Input: part model. Units: mm. Frame: model coordinates. A direction names the side the tool comes from. Coordinates: 2 decimals unless noted, no trailing zeros. Write each loop counter-clockwise with the first axis right and the second up, starting at its lowest first coordinate (ties: lowest second). Pieces come first, ordered by that corner, then holes.
1) Section query B-B (x = -119). Output: boundary loops of the cut face in (y, z).
2) Set-up query: faces 1 (the flat face through (-35, 19, -50)), 2 (the flat face through (-83, 7, 23)), 3 (the flat face through (-240, 19, -25.991)), 4 (the flat face through (-240, 19, 124.009)). Return all of +Z, -Z, +X, -X, +Y, -Y with unobstructed straight access to the full face (end or side cutting, diameter ignored); none if empty.
3) Pin query (flat end, axial travel): pin 1 Ø1.5 at (x, y) = (-18, 20) entering from +Z; pin 2 Ø1.6 at (y, z) = (6.5, -4) entering from +X; pin 3 Ø7.5 at (y, z) = (25.5, -47) entering from -X. Return the tip coordinate at first contact, or that it passes through.
4) Draft query along Y for faces 5 (the flat face through (-240, 32, 99)), 6 (the flat face through (-243, 7, 73)), 7 (the flat face through (-80, 19, 75.261)). Return one class per face: pulls with the +Y half, pulls with the -Y half, needs draft (parallel to the pull), parting line crosses it, or undercut.
5) Section query A-A (y = 16.5). State how many separate pieces and enclosed holes the cut face has, then the cut area to 3 significant figures.
6) Line query: L1, parallel to X at y = 27.5, z = 55; L2, parallel to Z at x = 5.5, y = 20.5. Output: solid intervals per line, ascending.
from build123d import *

# Parameters (mm, degrees)
SKETCH1_W                  = 80
SKETCH1_H                  = 270
BOSS_EXTRUDE1_DEPTH        = 5
SKETCH2_W                  = 65
SKETCH2_H                  = 45
BOSS_EXTRUDE3_DEPTH        = 2
LPATTERN1_COUNT            = 5
LPATTERN1_PITCH            = 50
SKETCH3_W                  = 70
SKETCH3_H                  = 48.748964222
BOSS_EXTRUDE8_DEPTH        = 25
LPATTERN5_COUNT            = 5
LPATTERN5_PITCH            = 50
LPATTERN6_COUNT            = 4
LPATTERN6_PITCH            = 80
LPATTERN6_COPY_1_SKETCH_W  = 65
LPATTERN6_COPY_1_SKETCH_H  = 45
LPATTERN6_COPY_1_DEPTH     = 2
LPATTERN6_COPY_2_SKETCH_W  = 65
LPATTERN6_COPY_2_SKETCH_H  = 45
LPATTERN6_COPY_2_DEPTH     = 2
LPATTERN6_COPY_3_SKETCH_W  = 65
LPATTERN6_COPY_3_SKETCH_H  = 45
LPATTERN6_COPY_3_DEPTH     = 2
LPATTERN6_COPY_4_SKETCH_W  = 65
LPATTERN6_COPY_4_SKETCH_H  = 45
LPATTERN6_COPY_4_DEPTH     = 2
LPATTERN6_COPY_5_SKETCH_W  = 65
LPATTERN6_COPY_5_SKETCH_H  = 45
LPATTERN6_COPY_5_DEPTH     = 2
LPATTERN6_COPY_6_SKETCH_W  = 65
LPATTERN6_COPY_6_SKETCH_H  = 45
LPATTERN6_COPY_6_DEPTH     = 2
LPATTERN6_COPY_7_SKETCH_W  = 65
LPATTERN6_COPY_7_SKETCH_H  = 45
LPATTERN6_COPY_7_DEPTH     = 2
LPATTERN6_COPY_8_SKETCH_W  = 65
LPATTERN6_COPY_8_SKETCH_H  = 45
LPATTERN6_COPY_8_DEPTH     = 2
LPATTERN6_COPY_9_SKETCH_W  = 65
LPATTERN6_COPY_9_SKETCH_H  = 45
LPATTERN6_COPY_9_DEPTH     = 2
LPATTERN6_COPY_10_SKETCH_W = 65
LPATTERN6_COPY_10_SKETCH_H = 45
LPATTERN6_COPY_10_DEPTH    = 2
LPATTERN6_COPY_11_SKETCH_W = 65
LPATTERN6_COPY_11_SKETCH_H = 45
LPATTERN6_COPY_11_DEPTH    = 2
LPATTERN6_COPY_12_SKETCH_W = 65
LPATTERN6_COPY_12_SKETCH_H = 45
LPATTERN6_COPY_12_DEPTH    = 2
LPATTERN6_COPY_13_SKETCH_W = 70
LPATTERN6_COPY_13_SKETCH_H = 48.748964222
LPATTERN6_COPY_13_DEPTH    = 25
LPATTERN6_COPY_14_SKETCH_W = 70
LPATTERN6_COPY_14_SKETCH_H = 48.748964222
LPATTERN6_COPY_14_DEPTH    = 25
LPATTERN6_COPY_15_SKETCH_W = 70
LPATTERN6_COPY_15_SKETCH_H = 48.748964222
LPATTERN6_COPY_15_DEPTH    = 25
LPATTERN6_COPY_16_SKETCH_W = 70
LPATTERN6_COPY_16_SKETCH_H = 48.748964222
LPATTERN6_COPY_16_DEPTH    = 25
LPATTERN6_COPY_17_SKETCH_W = 70
LPATTERN6_COPY_17_SKETCH_H = 48.748964222
LPATTERN6_COPY_17_DEPTH    = 25
LPATTERN6_COPY_18_SKETCH_W = 70
LPATTERN6_COPY_18_SKETCH_H = 48.748964222
LPATTERN6_COPY_18_DEPTH    = 25
LPATTERN6_COPY_19_SKETCH_W = 70
LPATTERN6_COPY_19_SKETCH_H = 48.748964222
LPATTERN6_COPY_19_DEPTH    = 25
LPATTERN6_COPY_20_SKETCH_W = 70
LPATTERN6_COPY_20_SKETCH_H = 48.748964222
LPATTERN6_COPY_20_DEPTH    = 25
LPATTERN6_COPY_21_SKETCH_W = 70
LPATTERN6_COPY_21_SKETCH_H = 48.748964222
LPATTERN6_COPY_21_DEPTH    = 25
LPATTERN6_COPY_22_SKETCH_W = 70
LPATTERN6_COPY_22_SKETCH_H = 48.748964222
LPATTERN6_COPY_22_DEPTH    = 25
LPATTERN6_COPY_23_SKETCH_W = 70
LPATTERN6_COPY_23_SKETCH_H = 48.748964222
LPATTERN6_COPY_23_DEPTH    = 25
LPATTERN6_COPY_24_SKETCH_W = 70
LPATTERN6_COPY_24_SKETCH_H = 48.748964222
LPATTERN6_COPY_24_DEPTH    = 25


with BuildPart() as part:
    # Sketch1 → Boss-Extrude1 (new body)
    with BuildSketch(Plane(origin=(0, 0, 0), x_dir=(1, 0, 0), z_dir=(0, 1, 0))):
        Rectangle(SKETCH1_W, SKETCH1_H)
    boss_extrude1 = extrude(amount=BOSS_EXTRUDE1_DEPTH)

    # Sketch2 → Boss-Extrude3 (add)
    with BuildSketch(Plane(origin=(0, 5, 0), x_dir=(1, 0, 0), z_dir=(0, 1, 0))):
        with Locations((0, -100)):
            Rectangle(SKETCH2_W, SKETCH2_H)
    boss_extrude3 = extrude(amount=BOSS_EXTRUDE3_DEPTH)

    # LPattern1: Boss-Extrude3 ×5
    with Locations(*[(0, 0, -i * LPATTERN1_PITCH) for i in range(1, LPATTERN1_COUNT)]):
        add(boss_extrude3)

    # Sketch3 → Boss-Extrude8 (add)
    with BuildSketch(Plane(origin=(0, 7, 0), x_dir=(1, 0, 0), z_dir=(0, 1, 0))):
        with Locations((0, -99.635002086)):
            Rectangle(SKETCH3_W, SKETCH3_H)
    boss_extrude8 = extrude(amount=BOSS_EXTRUDE8_DEPTH)

    # LPattern5: Boss-Extrude8 ×5
    with Locations(*[(0, 0, -i * LPATTERN5_PITCH) for i in range(1, LPATTERN5_COUNT)]):
        add(boss_extrude8)

    # LPattern6: Boss-Extrude1, Boss-Extrude3, Boss-Extrude8 ×4
    with Locations(*[(-i * LPATTERN6_PITCH, 0, 0) for i in range(1, LPATTERN6_COUNT)]):
        add(boss_extrude1)
        add(boss_extrude3)
        add(boss_extrude8)

    # LPattern6 copy 1 sketch → LPattern6 copy 1 (add)
    with BuildSketch(Plane(origin=(-80, 5, -50), x_dir=(1, 0, 0), z_dir=(0, 1, 0))):
        with Locations((0, -100)):
            Rectangle(LPATTERN6_COPY_1_SKETCH_W, LPATTERN6_COPY_1_SKETCH_H)
    extrude(amount=LPATTERN6_COPY_1_DEPTH)

    # LPattern6 copy 2 sketch → LPattern6 copy 2 (add)
    with BuildSketch(Plane(origin=(-160, 5, -50), x_dir=(1, 0, 0), z_dir=(0, 1, 0))):
        with Locations((0, -100)):
            Rectangle(LPATTERN6_COPY_2_SKETCH_W, LPATTERN6_COPY_2_SKETCH_H)
    extrude(amount=LPATTERN6_COPY_2_DEPTH)

    # LPattern6 copy 3 sketch → LPattern6 copy 3 (add)
    with BuildSketch(Plane(origin=(-240, 5, -50), x_dir=(1, 0, 0), z_dir=(0, 1, 0))):
        with Locations((0, -100)):
            Rectangle(LPATTERN6_COPY_3_SKETCH_W, LPATTERN6_COPY_3_SKETCH_H)
    extrude(amount=LPATTERN6_COPY_3_DEPTH)

    # LPattern6 copy 4 sketch → LPattern6 copy 4 (add)
    with BuildSketch(Plane(origin=(-80, 5, -100), x_dir=(1, 0, 0), z_dir=(0, 1, 0))):
        with Locations((0, -100)):
            Rectangle(LPATTERN6_COPY_4_SKETCH_W, LPATTERN6_COPY_4_SKETCH_H)
    extrude(amount=LPATTERN6_COPY_4_DEPTH)

    # LPattern6 copy 5 sketch → LPattern6 copy 5 (add)
    with BuildSketch(Plane(origin=(-160, 5, -100), x_dir=(1, 0, 0), z_dir=(0, 1, 0))):
        with Locations((0, -100)):
            Rectangle(LPATTERN6_COPY_5_SKETCH_W, LPATTERN6_COPY_5_SKETCH_H)
    extrude(amount=LPATTERN6_COPY_5_DEPTH)

    # LPattern6 copy 6 sketch → LPattern6 copy 6 (add)
    with BuildSketch(Plane(origin=(-240, 5, -100), x_dir=(1, 0, 0), z_dir=(0, 1, 0))):
        with Locations((0, -100)):
            Rectangle(LPATTERN6_COPY_6_SKETCH_W, LPATTERN6_COPY_6_SKETCH_H)
    extrude(amount=LPATTERN6_COPY_6_DEPTH)

    # LPattern6 copy 7 sketch → LPattern6 copy 7 (add)
    with BuildSketch(Plane(origin=(-80, 5, -150), x_dir=(1, 0, 0), z_dir=(0, 1, 0))):
        with Locations((0, -100)):
            Rectangle(LPATTERN6_COPY_7_SKETCH_W, LPATTERN6_COPY_7_SKETCH_H)
    extrude(amount=LPATTERN6_COPY_7_DEPTH)

    # LPattern6 copy 8 sketch → LPattern6 copy 8 (add)
    with BuildSketch(Plane(origin=(-160, 5, -150), x_dir=(1, 0, 0), z_dir=(0, 1, 0))):
        with Locations((0, -100)):
            Rectangle(LPATTERN6_COPY_8_SKETCH_W, LPATTERN6_COPY_8_SKETCH_H)
    extrude(amount=LPATTERN6_COPY_8_DEPTH)

    # LPattern6 copy 9 sketch → LPattern6 copy 9 (add)
    with BuildSketch(Plane(origin=(-240, 5, -150), x_dir=(1, 0, 0), z_dir=(0, 1, 0))):
        with Locations((0, -100)):
            Rectangle(LPATTERN6_COPY_9_SKETCH_W, LPATTERN6_COPY_9_SKETCH_H)
    extrude(amount=LPATTERN6_COPY_9_DEPTH)

    # LPattern6 copy 10 sketch → LPattern6 copy 10 (add)
    with BuildSketch(Plane(origin=(-80, 5, -200), x_dir=(1, 0, 0), z_dir=(0, 1, 0))):
        with Locations((0, -100)):
            Rectangle(LPATTERN6_COPY_10_SKETCH_W, LPATTERN6_COPY_10_SKETCH_H)
    extrude(amount=LPATTERN6_COPY_10_DEPTH)

    # LPattern6 copy 11 sketch → LPattern6 copy 11 (add)
    with BuildSketch(Plane(origin=(-160, 5, -200), x_dir=(1, 0, 0), z_dir=(0, 1, 0))):
        with Locations((0, -100)):
            Rectangle(LPATTERN6_COPY_11_SKETCH_W, LPATTERN6_COPY_11_SKETCH_H)
    extrude(amount=LPATTERN6_COPY_11_DEPTH)

    # LPattern6 copy 12 sketch → LPattern6 copy 12 (add)
    with BuildSketch(Plane(origin=(-240, 5, -200), x_dir=(1, 0, 0), z_dir=(0, 1, 0))):
        with Locations((0, -100)):
            Rectangle(LPATTERN6_COPY_12_SKETCH_W, LPATTERN6_COPY_12_SKETCH_H)
    extrude(amount=LPATTERN6_COPY_12_DEPTH)

    # LPattern6 copy 13 sketch → LPattern6 copy 13 (add)
    with BuildSketch(Plane(origin=(-80, 7, -50), x_dir=(1, 0, 0), z_dir=(0, 1, 0))):
        with Locations((0, -99.635002086)):
            Rectangle(LPATTERN6_COPY_13_SKETCH_W, LPATTERN6_COPY_13_SKETCH_H)
    extrude(amount=LPATTERN6_COPY_13_DEPTH)

    # LPattern6 copy 14 sketch → LPattern6 copy 14 (add)
    with BuildSketch(Plane(origin=(-160, 7, -50), x_dir=(1, 0, 0), z_dir=(0, 1, 0))):
        with Locations((0, -99.635002086)):
            Rectangle(LPATTERN6_COPY_14_SKETCH_W, LPATTERN6_COPY_14_SKETCH_H)
    extrude(amount=LPATTERN6_COPY_14_DEPTH)

    # LPattern6 copy 15 sketch → LPattern6 copy 15 (add)
    with BuildSketch(Plane(origin=(-240, 7, -50), x_dir=(1, 0, 0), z_dir=(0, 1, 0))):
        with Locations((0, -99.635002086)):
            Rectangle(LPATTERN6_COPY_15_SKETCH_W, LPATTERN6_COPY_15_SKETCH_H)
    extrude(amount=LPATTERN6_COPY_15_DEPTH)

    # LPattern6 copy 16 sketch → LPattern6 copy 16 (add)
    with BuildSketch(Plane(origin=(-80, 7, -100), x_dir=(1, 0, 0), z_dir=(0, 1, 0))):
        with Locations((0, -99.635002086)):
            Rectangle(LPATTERN6_COPY_16_SKETCH_W, LPATTERN6_COPY_16_SKETCH_H)
    extrude(amount=LPATTERN6_COPY_16_DEPTH)

    # LPattern6 copy 17 sketch → LPattern6 copy 17 (add)
    with BuildSketch(Plane(origin=(-160, 7, -100), x_dir=(1, 0, 0), z_dir=(0, 1, 0))):
        with Locations((0, -99.635002086)):
            Rectangle(LPATTERN6_COPY_17_SKETCH_W, LPATTERN6_COPY_17_SKETCH_H)
    extrude(amount=LPATTERN6_COPY_17_DEPTH)

    # LPattern6 copy 18 sketch → LPattern6 copy 18 (add)
    with BuildSketch(Plane(origin=(-240, 7, -100), x_dir=(1, 0, 0), z_dir=(0, 1, 0))):
        with Locations((0, -99.635002086)):
            Rectangle(LPATTERN6_COPY_18_SKETCH_W, LPATTERN6_COPY_18_SKETCH_H)
    extrude(amount=LPATTERN6_COPY_18_DEPTH)

    # LPattern6 copy 19 sketch → LPattern6 copy 19 (add)
    with BuildSketch(Plane(origin=(-80, 7, -150), x_dir=(1, 0, 0), z_dir=(0, 1, 0))):
        with Locations((0, -99.635002086)):
            Rectangle(LPATTERN6_COPY_19_SKETCH_W, LPATTERN6_COPY_19_SKETCH_H)
    extrude(amount=LPATTERN6_COPY_19_DEPTH)

    # LPattern6 copy 20 sketch → LPattern6 copy 20 (add)
    with BuildSketch(Plane(origin=(-160, 7, -150), x_dir=(1, 0, 0), z_dir=(0, 1, 0))):
        with Locations((0, -99.635002086)):
            Rectangle(LPATTERN6_COPY_20_SKETCH_W, LPATTERN6_COPY_20_SKETCH_H)
    extrude(amount=LPATTERN6_COPY_20_DEPTH)

    # LPattern6 copy 21 sketch → LPattern6 copy 21 (add)
    with BuildSketch(Plane(origin=(-240, 7, -150), x_dir=(1, 0, 0), z_dir=(0, 1, 0))):
        with Locations((0, -99.635002086)):
            Rectangle(LPATTERN6_COPY_21_SKETCH_W, LPATTERN6_COPY_21_SKETCH_H)
    extrude(amount=LPATTERN6_COPY_21_DEPTH)

    # LPattern6 copy 22 sketch → LPattern6 copy 22 (add)
    with BuildSketch(Plane(origin=(-80, 7, -200), x_dir=(1, 0, 0), z_dir=(0, 1, 0))):
        with Locations((0, -99.635002086)):
            Rectangle(LPATTERN6_COPY_22_SKETCH_W, LPATTERN6_COPY_22_SKETCH_H)
    extrude(amount=LPATTERN6_COPY_22_DEPTH)

    # LPattern6 copy 23 sketch → LPattern6 copy 23 (add)
    with BuildSketch(Plane(origin=(-160, 7, -200), x_dir=(1, 0, 0), z_dir=(0, 1, 0))):
        with Locations((0, -99.635002086)):
            Rectangle(LPATTERN6_COPY_23_SKETCH_W, LPATTERN6_COPY_23_SKETCH_H)
    extrude(amount=LPATTERN6_COPY_23_DEPTH)

    # LPattern6 copy 24 sketch → LPattern6 copy 24 (add)
    with BuildSketch(Plane(origin=(-240, 7, -200), x_dir=(1, 0, 0), z_dir=(0, 1, 0))):
        with Locations((0, -99.635002086)):
            Rectangle(LPATTERN6_COPY_24_SKETCH_W, LPATTERN6_COPY_24_SKETCH_H)
    extrude(amount=LPATTERN6_COPY_24_DEPTH)


solid = part.part
Answer:
1. outline: (0, -135) - (5, -135) - (5, 135) - (0, 135) - close
2. face 1: +Z, -Z, +Y
2. face 2: none
2. face 3: +X, -X, +Y
2. face 4: +Z, +X, -X, +Y
3. pin 1: stops at z = 124.01
3. pin 2: stops at x = 35
3. pin 3: stops at x = -275
4. face 5: pulls with the +Y half
4. face 6: undercut
4. face 7: needs draft
5. separate pieces: 20
5. enclosed holes: 0
5. area: 68,200 mm2
6. L1: x = -275 to -205, -195 to -125, -115 to -45, -35 to 35
6. L2: z = -124.74 to -75.99, -74.74 to -25.99, -24.74 to 24.01, 25.26 to 74.01, 75.26 to 124.01
